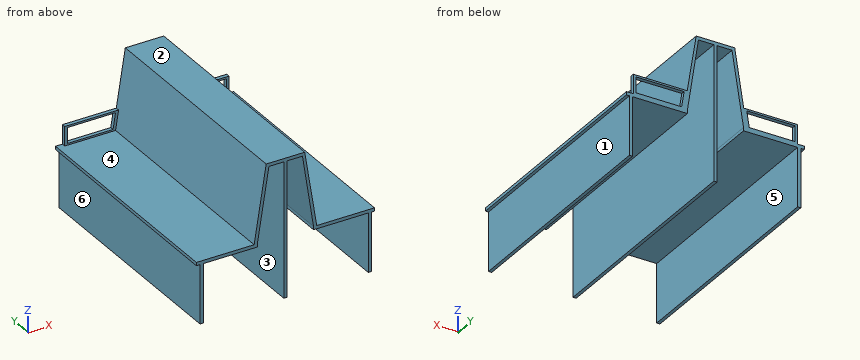
from build123d import *

# Parameters (mm, degrees)
F0_W     = 25.4
F0_H     = 464.7051875732
F0_H_2   = 1066.8
F0_H_3   = 25.4
F1_DEPTH = 1828.8
F2_DEPTH = 30


# Not quite as in the source:
# - a feature names something its author has since deleted; it is built from what else it names


with BuildPart() as f1:
    # F0 (on Front) → F1 (new body)
    with BuildSketch(Plane.XZ):
        with Locations((-415.2822112945, -802.4841870543)):
            Rectangle(F0_W, F0_H)
        with Locations((247.7624498885, -501.4367808409)):
            Rectangle(F0_W, F0_H_2)
        with Locations((915.8871110716, -802.4841870543)):
            Rectangle(F0_W, F0_H)
        with Locations((12.7, -557.4315932677)):
            Rectangle(F0_W, F0_H_3)
        Polygon((145.9203362465, 57.3632191591), (95.3624498885, 57.3632191591), (24.1377887055, -392.3315932677), (0, -544.7315932677), (25.4, -544.7315932677), (116.7394851043, 31.9632191591), (145.9203362465, 31.9632191591), align=None)
        Polygon((362.7394139767, 57.3632191591), (145.9203362465, 57.3632191591), (145.9203362465, 31.9632191591), (235.0624498885, 31.9632191591), (260.4624498885, 31.9632191591), (362.7394139767, 31.9632191591), align=None)
        Polygon((898.1071110716, -544.7315932677), (495.524899777, -544.7315932677), (470.124899777, -544.7315932677), (470.124899777, -570.1315932677), (903.1871110716, -570.1315932677), (928.5871110716, -570.1315932677), (952.7248997771, -570.1315932677), (952.724899777, -544.7315932677), align=None)
        Polygon((400.1624498885, 57.3632191591), (362.7394139767, 57.3632191591), (362.7394139767, 31.9632191591), (382.4598755032, 31.9632191591), (470.124899777, -544.7315932677), (495.524899777, -544.7315932677), (471.3871110716, -392.3315932677), align=None)
        Polygon((0, -570.1315932677), (0, -544.7315932677), (-402.5822112945, -544.7315932677), (-457.2, -544.7315932677), (-457.2, -570.1315932677), (-427.9822112945, -570.1315932677), (-402.5822112945, -570.1315932677), align=None)
    extrude(amount=F1_DEPTH)

    # F0 (on Front) → F2 (join)
    with BuildSketch(Plane.XZ):
        Polygon((0, -544.7315932677), (24.1377887055, -392.3315932677), (-402.5822112945, -392.3315932677), (-402.5822112945, -544.7315932677), align=None)
        Polygon((-382.1481764317, -406.8649113178), (0, -406.0111343861), (-19.8426051641, -531.2924127962), (-382.1481764317, -531.2924127962), align=None, mode=Mode.SUBTRACT)
        Polygon((898.1071110716, -392.3315932677), (471.3871110716, -392.3315932677), (495.524899777, -544.7315932677), (898.1071110716, -544.7315932677), align=None)
        Polygon((495.524899777, -406.0111343861), (877.6730762087, -406.8649113178), (877.6730762087, -531.2924127962), (515.3675049412, -531.2924127962), align=None, mode=Mode.SUBTRACT)
    extrude(amount=F2_DEPTH)


solid = f1.part
Verification items for the finished model (mm, model axes). Face numbers are marked on the shaded views. A direction names the side the tool comes from. Give positions to 0.01 mm unless a question says otherwise; leave off trailing zeros. Loops run counter-clockwise (first coordinate to the right, second up) from the corner with the lowest first, then second, coordinate; pieces in that order, holes last.
1) Set-up check for the marked faces 1, 2 and 3: record each of +Z, -Z, +X, -X, +Y, -Y from which the full face is reachable in a straight line by a thin tool's end or side.
2) Draft check along X on the marked faces 4, 5 and 6. Enter one of: pulls with the +X half, pulls with the -X half, needs draft (parallel to the pull), parting line crosses it, or undercut.
3) Depth check by flat-ended pin: pin 1 Ø3 at (y, z) = (-1468, -907.5) entering from +X; pin 2 Ø9 at (x, y) = (-193.5, -11.5) entering from +Z; pin 3 Ø2 at (x, y) = (165, -928) entering from -Z. Enter the tip coordinate at first touch or a pass-through.
4) Sectioned sample at D-D, the plane z = -501. Enter the section's corners in (x, y), then the cut area to 3 significant figures.
5) Thickness scan on line 1 along X through (y, z) = (-1205.5, -906); line 2 along X through (y, z) = (-1480, -200.5); line 3 along Z through (x, y) = (162.5, -125.5). Record the ranges inside material, lowest first.
6) Sectioned sample at C-C, the plane y = -1335. Enter the section's corners in (x, z).
7) Sectioned sample at B-B, the plane x = -217.5. Enter the section's corners in (y, z).
8) Sectioned sample at A-A, the plane z = -811.5. Enter the section's corners in (x, y).
Answers:
1. face 1: -Z, +X, +Y, -Y
1. face 2: +Z, +X, -X, +Y, -Y
1. face 3: -Z, +Y, -Y
2. face 4: needs draft
2. face 5: undercut
2. face 6: pulls with the -X half
3. pin 1: stops at x = 928.59
3. pin 2: stops at z = -392.33
3. pin 3: stops at z = 31.96
4. outline: (-402.58, -30) - (-382.15, -30) - (-382.15, 0) - (-402.58, 0) - close; (-15.04, -30) - (6.93, -30) - (6.93, -1828.8) - (32.33, -1828.8) - (32.33, 0) - (-15.04, 0) - close; (235.06, -1828.8) - (260.46, -1828.8) - (260.46, 0) - (235.06, 0) - close; (463.48, -1828.8) - (488.6, -1828.8) - (488.6, -30) - (510.57, -30) - (510.57, 0) - (463.48, 0) - close; (877.67, -30) - (898.11, -30) - (898.11, 0) - (877.67, 0) - close
4. area: 141,000 mm2
5. line 1: x = -427.98 to -402.58, 235.06 to 260.46, 903.19 to 928.59
5. line 2: x = 54.52 to 79.92, 235.06 to 260.46, 417.8 to 441
5. line 3: z = 31.96 to 57.36
6. outline: (-457.2, -570.13) - (-427.98, -570.13) - (-427.98, -1034.84) - (-402.58, -1034.84) - (-402.58, -570.13) - (25.4, -570.13) - (25.4, -544.73) - (116.74, 31.96) - (235.06, 31.96) - (235.06, -1034.84) - (260.46, -1034.84) - (260.46, 31.96) - (382.46, 31.96) - (470.12, -544.73) - (470.12, -570.13) - (903.19, -570.13) - (903.19, -1034.84) - (928.59, -1034.84) - (928.59, -570.13) - (952.72, -570.13) - (952.72, -544.73) - (495.52, -544.73) - (400.16, 57.36) - (95.36, 57.36) - (0, -544.73) - (-457.2, -544.73) - close
7. outline: (-1828.8, -570.13) - (0, -570.13) - (0, -531.29) - (-30, -531.29) - (-30, -544.73) - (-1828.8, -544.73) - close; (-30, -406.5) - (0, -406.5) - (0, -392.33) - (-30, -392.33) - close
8. outline: (-427.98, -1828.8) - (-402.58, -1828.8) - (-402.58, 0) - (-427.98, 0) - close; (235.06, -1828.8) - (260.46, -1828.8) - (260.46, 0) - (235.06, 0) - close; (903.19, -1828.8) - (928.59, -1828.8) - (928.59, 0) - (903.19, 0) - close
